Autodesk Inventor part; units mm, degrees
ref_plane "YZ Plane" through (0, 0, 0) normal (1, 0, 0) x (0, 1, 0)
ref_plane "XZ Plane" through (0, 0, 0) normal (0, 1, 0) x (-1, 0, 0)
ref_plane "XY Plane" through (0, 0, 0) normal (0, 0, 1) x (1, 0, 0)
sketch "スケッチ1" plane through (0, 0, 0) normal (0, 0, 1) x (1, 0, 0)
  line L0 (0, 0) -> (14, 0)
  line L1 (14, 0) -> (14, 117)
  line L2 (14, 117) -> (0, 117)
  line L3 (0, 117) -> (0, 109.16)
  line L4 (0, 109.16) -> (3.5, 109.16)
  line L5 (3.5, 109.16) -> (3.5, 7.84)
  line L6 (3.5, 7.84) -> (0, 7.84)
  line L7 (0, 7.84) -> (0, 0)
  dimension "d0" = 117
  dimension "d1" = 3.5
  dimension "d2" = 7.84
  dimension "d3" = 14
extrude "押し出し1" add sketch "スケッチ1" along normal blind 14.4
sketch "スケッチ2" plane through (0, 0, 0) normal (-1, 0, 0) x (0, 0, 1)
  line L0 (0, 117) -> (14.4, 117) construction
  line L1 (0, 0) -> (14.4, 0) construction
  line L2 (0, 117) -> (14.4, 117) construction
  line L3 (7.15, 117) -> (7.15, 0) construction
  line L4 (0, 0) -> (14.4, 0) construction
  circle A0 centre (7.15, 4.35) radius 1.8 construction
  line L5 (7.15, 4.35) -> (5.35, 4.35) construction
  line L6 (0, 7.84) -> (0, 0) construction
  circle A1 centre (7.15, 4.35) radius 2.25
  line L7 (7.15, 58.5) -> (14.4, 58.5) construction
  line L8 (14.4, 0) -> (14.4, 117)
  circle A2 centre (7.15, 112.65) radius 2.25
  point P0 (7.15, 2.55)
  dimension "d6" = 3.6
  dimension "d7" = 5.35
  dimension "d8" = 2.55
  dimension "d9" = 4.5
extrude "押し出し2" cut sketch "スケッチ2" against normal through all
fillet "フィレット1" radius 5 2 edges at (7, 0, 14.4) (7, 117, 14.4)
sketch "スケッチ3" plane through (0, 0, 0) normal (0, 0, -1) x (-1, 0, 0)
  line L0 (0, 7.84) -> (0, 0) construction
  line L1 (-14, 0) -> (-14, 117) construction
  line L2 (0, 117) -> (0, 109.16) construction
  line L3 (0, 3.92) -> (-14, 3.92) construction
  circle A0 centre (-10, 3.92) radius 2.25
  line L4 (-14, 5) -> (-14, 112) construction
  line L5 (-14, 58.5) -> (-3.7036, 58.5) construction
  circle A1 centre (-10, 113.08) radius 2.25
  dimension "d13" = 7.84
  dimension "d14" = 4.5
  dimension "d17" = 4
extrude "押し出し3" cut sketch "スケッチ3" against normal blind 7.5
fillet "フィレット2" radius 4 5 edges at (14, 1.4645, 12.9355) (14, 58.5, 14.4) (14, 115.5355, 12.9355) (14, 117, 4.7) (14, 0, 4.7)
properties part number "small_gpu_03" material "アルミニウム 6061"
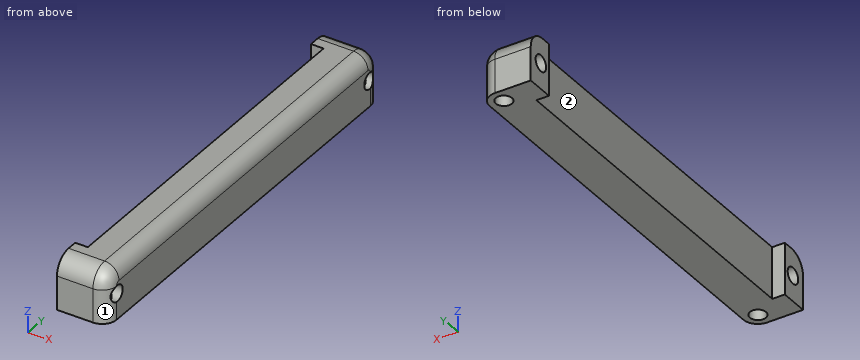
Here's how the part is built. I have some questions about the finished solid (model axes, mm). Face numbers are marked on the shaded views. A direction names the side the tool comes from. Give positions to 0.01 mm unless a question says otherwise; leave off trailing zeros. Write each loop counter-clockwise with the first axis right and the second up, starting at its lowest first coordinate (ties: lowest second). Pieces come first, ordered by that corner, then holes.
(1) If I drill on L1, parallel to Y at x = 10.25, z = 1.5; L2, parallel to Y at x = 3, z = 7.15; L3, parallel to Y at x = 7.75, z = 7.15, over which ranges is the centre line in solid material (lowest first)?
Output values:
L1: y = 0.01 to 1.68, 6.16 to 110.84, 115.32 to 116.99
L2: y = 0 to 2.1, 6.6 to 7.84, 109.16 to 110.4, 114.9 to 117
L3: y = 0 to 2.1, 6.6 to 110.4, 114.9 to 117
(2) Will this pin go through, and if not, where does the flat tip stop? pin 1 (4 mm diameter, centred on x = 1.5, z = 13, fed in from -Y).
Output values:
pin 1: stops at y = 0.26
(3) On a 3-axis mill with a long thin cutter (end or side, diameter ignored), from which of +Z, -Z, +X, -X, +Y, -Y can I reach the whole of each face in a straight line? I mean the marked faces 1 and 2. Say none if no direction works.
Output values:
face 1: +Z, -Z, +X, -Y
face 2: +Z, -Z, -X
(4) Imagine slicing it at C-C, the plane y = 101.5. Write out the boundary of the cut face in (x, z).
Output values:
outline: (3.5, 0) - (14, 0) - (14, 10.4) arc R4 ccw to (10, 14.4) - (3.5, 14.4) - close
(5) Imagine slicing it at A-A, the plane x = 2.5. Write out the boundary of the cut face in (y, z).
Output values:
outline: (0, 0) - (7.84, 0) - (7.84, 14.4) - (5, 14.4) arc R5 ccw to (0, 9.4) - close; (109.16, 0) - (117, 0) - (117, 9.4) arc R5 ccw to (112, 14.4) - (109.16, 14.4) - close; hole circle Ø4.5 at (4.35, 7.15); hole circle Ø4.5 at (112.65, 7.15)
(6) Imagine slicing it at B-B, the plane z = 3.75. Write out the boundary of the cut face in (x, y), and give its area (3 significant figures).
Output values:
outline: (0, 0) - (10, 0) arc R4 ccw to (14, 4) - (14, 113) arc R4 ccw to (10, 117) - (0, 117) - (0, 109.16) - (3.5, 109.16) - (3.5, 7.84) - (0, 7.84) - close; hole circle Ø4.5 at (10, 3.92); hole circle Ø4.5 at (10, 113.08)
area: 1,240 mm2
